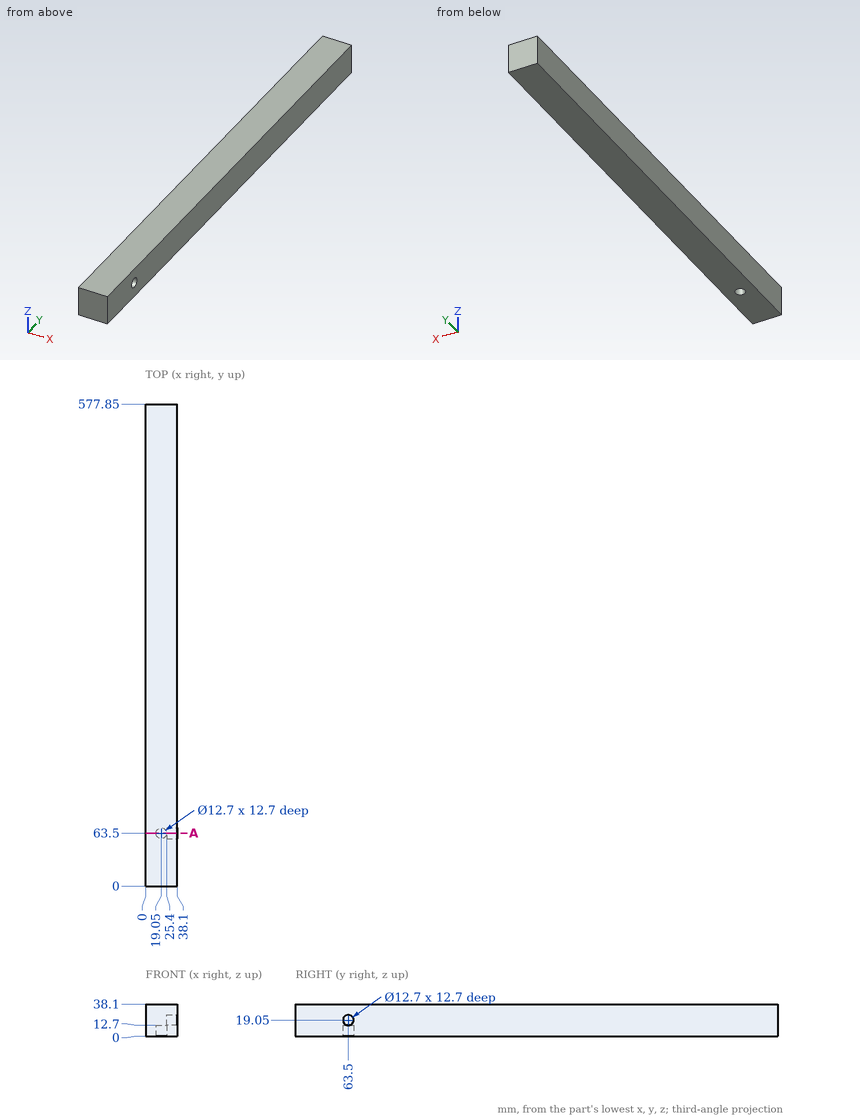
Geometry: see drawing. Coordinates: mm, zero at the bounding-box minimum. Round coordinates to 2 decimals unless told otherwise and drop trailing zeros. Write each loop counter-clockwise with the first axis right and the second up, starting at its lowest first coordinate (ties: lowest second). Pieces come first, ordered by that corner, then holes. Notation, with made-up numbers: M 2.5,61.25 L 59.5,61.25 A28 ccw 59.5,96.25 Z; hole C 25.5,-36.75 d2. An arc over 180 degrees is marked long. Answer as a JSON object with one key per item and string values. Group by question number.
(1) Section query A-A on y = 63.5. Output: boundary loops of the cut face in (x, z), then the cut area to 3 significant figures.
(2) Ray query, line 1 (Y direction, x = 19, z = 3); line 2 (Z direction, x = 28, y = 63); line 3 (Y direction, x = 24, z = 11). Return the intervals inside material, ascending. Write a range as [from, to].
(3) First-contact query: pin 1 (6.5 mm diameter, centred on y = 61, z = 20, fed in from +X); pin 2 (7.5 mm diameter, centred on x = 19.05, y = 63.5, fed in from -Z). Flat tips, straight axial feed; report the tip coordinate or a pass-through.
Computed values:
{
 "1": {"outline": "M 0,0 L 12.7,0 L 12.7,12.7 L 25.4,12.7 L 25.4,0 L 38.1,0 L 38.1,12.7 L 25.4,12.7 L 25.4,25.4 L 38.1,25.4 L 38.1,38.1 L 0,38.1 Z", "area": "1,130 mm^2"},
 "2": {"line 1": "[0, 57.15], [69.85, 577.85]", "line 2": "[0, 12.72], [25.38, 38.1]", "line 3": "[0, 59.52], [67.48, 577.85]"},
 "3": {"pin 1": "x = 25.4", "pin 2": "z = 12.7"}
}
